Input: part model. Units: mm. Frame: model coordinates. Round coordinates to 2 decimals unless told otherwise and drop trailing zeros. Loops run counter-clockwise (first coordinate to the right, second up) from the corner with the lowest first, then second, coordinate; pieces in that order, holes last. Notation, with made-up numbers: M 78.25,27 L 100.25,27 A18 ccw 100.25,61 Z; hole C -3,-32 d6. An arc over 180 degrees is marked long. Use one line per item in the form item = value. Start each with the question number.
Q1. Ray query, line 1 along X through (y, z) = (1.6, 0); line 2 along X through (y, z) = (2.15, -6); line 3 along Z through (x, y) = (50, 2.05). Return the intervals inside material, ascending.
Q2. Section query B-B, the plane z = 10. Output: boundary loops of the cut face in (x, y).
Q3. Section query C-C, the plane y = 1.1. State how many separate pieces and enclosed holes the cut face has, and give its area (3 significant figures).
Q4. Section query D-D, the plane x = 62.08. Output: boundary loops of the cut face in (y, z), and give its area (3 significant figures).
Q5. Section query A-A, the plane x = -28.73. Output: boundary loops of the cut face in (y, z).
```python
from build123d import *

# Parameters (mm, degrees)
BOSS_EXTRUDE1_DEPTH = 3.2
SKETCH2_W           = 10.76
SKETCH2_H           = 41.868700306
CUT_EXTRUDE1_DEPTH  = 103.580407486
SKETCH3_R           = 2
SKETCH3_R_2         = 2.25
CUT_EXTRUDE2_DEPTH  = 103.580407486
SKETCH4_R           = 15
CUT_EXTRUDE3_DEPTH  = 103.580407486
CUT_EXTRUDE4_DEPTH  = 103.580407486
SKETCH6_R           = 2.25
CUT_EXTRUDE5_DEPTH  = 103.580407486


with BuildPart() as part:
    # Sketch1 → Boss-Extrude1 (new body)
    with BuildSketch(Plane(origin=(0, 0, 0), x_dir=(1, 0, 0), z_dir=(0, 1, 0))):
        with BuildLine():
            ThreePointArc((33.29110537, -64.404598464), (0, 72.5), (-33.29110537, -64.404598464))
            ThreePointArc((-33.29110537, -64.404598464), (0, -44.989799638), (33.29110537, -64.404598464))
        make_face()
    extrude(amount=BOSS_EXTRUDE1_DEPTH)

    # Sketch2 → Cut-Extrude1 (cut, through all)
    with BuildSketch(Plane(origin=(0, 3.2, 0), x_dir=(1, 0, 0), z_dir=(0, 1, 0))):
        with Locations((-52.42, 0)):
            Rectangle(SKETCH2_W, SKETCH2_H)
        with Locations((52.42, 0)):
            Rectangle(SKETCH2_W, SKETCH2_H)
    extrude(amount=-CUT_EXTRUDE1_DEPTH, mode=Mode.SUBTRACT)

    # Sketch3 → Cut-Extrude2 (cut, through all)
    with BuildSketch(Plane.XZ):
        with Locations(Location((-62.08, 0, 0), (0, 0, 270))):
            Circle(SKETCH3_R)
        with Locations(Location((-28.73, 10, 0), (0, 0, 270))):
            Circle(SKETCH3_R_2)
        with Locations(Location((-28.73, -10, 0), (0, 0, 270))):
            Circle(SKETCH3_R_2)
        with Locations(Location((28.73, -10, 0), (0, 0, 90))):
            Circle(SKETCH3_R_2)
        with Locations(Location((28.73, 10, 0), (0, 0, 90))):
            Circle(SKETCH3_R_2)
        with Locations(Location((62.08, 0, 0), (0, 0, 90))):
            Circle(SKETCH3_R)
    extrude(amount=-CUT_EXTRUDE2_DEPTH, mode=Mode.SUBTRACT)

    # Sketch4 → Cut-Extrude3 (cut, through all)
    with BuildSketch(Plane(origin=(0, 3.2, 0), x_dir=(1, 0, 0), z_dir=(0, 1, 0))):
        with Locations(Location((-25, 48, 0), (0, 0, 270))):
            Circle(SKETCH4_R)
        with Locations(Location((25, 48, 0), (0, 0, 90))):
            Circle(SKETCH4_R)
    extrude(amount=-CUT_EXTRUDE3_DEPTH, mode=Mode.SUBTRACT)

    # Sketch5 → Cut-Extrude4 (cut, through all)
    with BuildSketch(Plane(origin=(0, 3.2, 0), x_dir=(1, 0, 0), z_dir=(0, 1, 0))):
        with BuildLine():
            Line((-56.385786438, 21.520136591), (-48.454213562, 21.520136591))
            ThreePointArc((-48.454213562, 21.520136591), (-47.04, 20.934350153), (-46.454213562, 19.520136591))
            Line((-46.454213562, 19.520136591), (-46.454213562, -19.520136591))
            ThreePointArc((-46.454213562, -19.520136591), (-47.04, -20.934350153), (-48.454213562, -21.520136591))
            Line((-48.454213562, -21.520136591), (-56.385786438, -21.520136591))
            ThreePointArc((-56.385786438, -21.520136591), (-57.8, -20.934350153), (-58.385786438, -19.520136591))
            Line((-58.385786438, -19.520136591), (-58.385786438, 19.520136591))
            ThreePointArc((-58.385786438, 19.520136591), (-57.8, 20.934350153), (-56.385786438, 21.520136591))
        make_face()
        with BuildLine():
            Line((46.454213562, 19.520136591), (46.454213562, -19.520136591))
            ThreePointArc((46.454213562, -19.520136591), (47.04, -20.934350153), (48.454213562, -21.520136591))
            Line((48.454213562, -21.520136591), (56.385786438, -21.520136591))
            ThreePointArc((56.385786438, -21.520136591), (57.8, -20.934350153), (58.385786438, -19.520136591))
            Line((58.385786438, -19.520136591), (58.385786438, 19.520136591))
            ThreePointArc((58.385786438, 19.520136591), (57.8, 20.934350153), (56.385786438, 21.520136591))
            Line((56.385786438, 21.520136591), (48.454213562, 21.520136591))
            ThreePointArc((48.454213562, 21.520136591), (47.04, 20.934350153), (46.454213562, 19.520136591))
        make_face()
    extrude(amount=-CUT_EXTRUDE4_DEPTH, mode=Mode.SUBTRACT)

    # Sketch6 → Cut-Extrude5 (cut, through all)
    with BuildSketch(Plane(origin=(0, 3.2, 0), x_dir=(1, 0, 0), z_dir=(0, 1, 0))):
        with Locations(Location((-50, 40, 0), (0, 0, 270))):
            Circle(SKETCH6_R)
        with Locations(Location((-35, -50, 0), (0, 0, 270))):
            Circle(SKETCH6_R)
        with Locations(Location((35, -50, 0), (0, 0, 90))):
            Circle(SKETCH6_R)
        with Locations(Location((50, 40, 0), (0, 0, 90))):
            Circle(SKETCH6_R)
    extrude(amount=-CUT_EXTRUDE5_DEPTH, mode=Mode.SUBTRACT)


solid = part.part
```
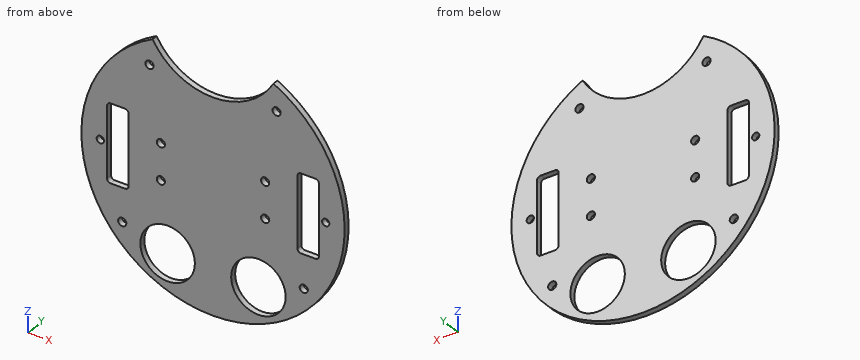
Results found:
q1.line_1 = -72.5 to -64.08, -60.08 to -58.39, -46.45 to 46.45, 58.39 to 60.08, 64.08 to 72.5
q1.line_2 = -72.25 to -58.39, -46.45 to 46.45, 58.39 to 72.25
q1.line_3 = -52.5 to -42.25, -37.75 to -21.52, 21.52 to 52.5
q2.outline = M -71.81,0 L -58.39,0 L -58.39,3.2 L -71.81,3.2 Z; M -46.45,0 L -30.98,0 L -30.98,3.2 L -46.45,3.2 Z; M -26.48,0 L 26.48,0 L 26.48,3.2 L -26.48,3.2 Z; M 30.98,0 L 46.45,0 L 46.45,3.2 L 30.98,3.2 Z; M 58.39,0 L 71.81,0 L 71.81,3.2 L 58.39,3.2 Z
q3.separate_pieces = 1
q3.enclosed_holes = 14
q3.area = 12,600 mm²
q4.outline = M 0,-37.45 L 3.2,-37.45 L 3.2,-2 L 0,-2 Z; M 0,2 L 3.2,2 L 3.2,37.45 L 0,37.45 Z
q4.area = 227 mm²
q5.outline = M 0,-66.56 L 3.2,-66.56 L 3.2,-62.53 L 0,-62.53 Z; M 0,-33.47 L 3.2,-33.47 L 3.2,-12.25 L 0,-12.25 Z; M 0,-7.75 L 3.2,-7.75 L 3.2,7.75 L 0,7.75 Z; M 0,12.25 L 3.2,12.25 L 3.2,57.99 L 0,57.99 Z
